from build123d import *

# Parameters (mm, degrees)
SKETCH2_W           = 46
SKETCH2_H           = 46
BOSS_EXTRUDE1_DEPTH = 5
SKETCH3_R           = 1.8
SKETCH3_R_2         = 2.5
CUT_EXTRUDE1_DEPTH  = 5
SKETCH4_R           = 4.1
CUT_EXTRUDE2_DEPTH  = 3
SKETCH5_W           = 4
SKETCH5_H           = 4
BOSS_EXTRUDE2_DEPTH = 3
SKETCH9_R           = 2
CUT_EXTRUDE6_DEPTH  = 6


with BuildPart() as part:
    # Sketch2 → Boss-Extrude1 (new body)
    with BuildSketch(Plane(origin=(0, 0, 0), x_dir=(1, 0, 0), z_dir=(0, 1, 0))):
        Rectangle(SKETCH2_W, SKETCH2_H)
    extrude(amount=BOSS_EXTRUDE1_DEPTH)

    # Sketch3 → Cut-Extrude1 (cut)
    with BuildSketch(Plane(origin=(0, 0, 0), x_dir=(1, 0, 0), z_dir=(0, 1, 0))):
        with Locations((-18.12, 19.125)):
            Circle(SKETCH3_R)
        with Locations((18.12, 19.125)):
            Circle(SKETCH3_R)
        with Locations((18.12, -19.125)):
            Circle(SKETCH3_R)
        with Locations((-18.12, -19.125)):
            Circle(SKETCH3_R)
        Circle(SKETCH3_R_2)
    extrude(amount=CUT_EXTRUDE1_DEPTH, mode=Mode.SUBTRACT)

    # Sketch4 → Cut-Extrude2 (cut)
    with BuildSketch(Plane(origin=(0, 0, 0), x_dir=(1, 0, 0), z_dir=(0, 1, 0))):
        Circle(SKETCH4_R)
    extrude(amount=CUT_EXTRUDE2_DEPTH, mode=Mode.SUBTRACT)

    # Sketch5 → Boss-Extrude2 (add)
    with BuildSketch(Plane(origin=(0, 0, 0), x_dir=(1, 0, 0), z_dir=(0, 1, 0))):
        with Locations((-5.7330026, 5.06948708)):
            Rectangle(SKETCH5_W, SKETCH5_H)
        with Locations((5.862376563, -4.939727226)):
            Rectangle(SKETCH5_W, SKETCH5_H)
    extrude(amount=-BOSS_EXTRUDE2_DEPTH)

    # Sketch9 → Cut-Extrude6 (cut, through all)
    with BuildSketch(Plane(origin=(0, 0, 0), x_dir=(1, 0, 0), z_dir=(0, 1, 0))):
        with Locations((-5.7330026, 20)):
            Circle(SKETCH9_R)
        with Locations((5.73, 20)):
            Circle(SKETCH9_R)
        with Locations((0, 20)):
            Circle(SKETCH9_R)
    extrude(amount=CUT_EXTRUDE6_DEPTH, mode=Mode.SUBTRACT)


solid = part.part
CAD build for the part. Positions are in the model's coordinates, mm. A direction names the side the tool comes from. Round coordinates to 2 decimals unless told otherwise and drop trailing zeros. Write each loop counter-clockwise with the first axis right and the second up, starting at its lowest first coordinate (ties: lowest second). Pieces come first, ordered by that corner, then holes. Notation, with made-up numbers: M -5.75,20 L 17.25,20 A21 cw 17.25,59 Z; hole C 18,23.25 d10. An arc over 180 degrees is marked long. Use a Markdown table: item, result. Add a question column.
1. Slice it at D-D on z = -1.5. Give the cut face in (x, y).
2. Drill centre lines: probe 1 along Z at (x, y) = (0, 1.85); probe 2 along X at (y, z) = (2, 0); probe 3 along Z at (x, y) = (-18.12, 1.55) (3 decimals). Where is each one in solid material? Low to high.
3. Slice it at A-A on x = 5.73. Give the cut face in (y, z).
4. Flat gauge pins, fed straight in: P1, Ø3, axis at x = 18.12, z = -19.125, coming from the -Y side; P2, Ø0.9, axis at x = -6.5, y = -1, coming from the -Z side; P3, Ø1.5, axis at y = -1, z = 5.5, coming from the +X side; P4, Ø0.9, axis at y = -1.5, z = -6, coming from the +X side. Where does each tip first touch, or does it go through?
5. Slice it at C-C on y = -2. Give the cut face in (x, z), then the cut area to 3 significant figures.
6. 3-axis set-ups, long thin cutter, end or side, ignore diameter. For faces 5 (the face through (6, -1, 2.94)), 6 (the face through (0, 2, 23)), 7 (the face through (-0.534, 1.479, -4.065)): which of +Z, -Z, +X, -X, +Y, -Y reach the whole face in a straight line?
7. Slice it at B-B on x = -18.12. Give the cut face in (y, z) (3 decimals).
8. Pull direction X, two halves, no side cores. Call faces 1 (the face through (7.862, -1, 5)), 2 (the face through (-2, 3, 2)), 3 (the face through (-7.733, -1, -5)), 4 (the face through (-6, -1, -7.069)): released by +X, released by -X, zero draft, split by the parting line, or undercut.
Reply:
| question | item | result |
|---|---|---|
| 1 | outline | M -23,0 L -3.82,0 L -3.82,3 L -2,3 L -2,5 L -23,5 Z; M 2,3 L 3.82,3 L 3.82,0 L 23,0 L 23,5 L 2,5 Z |
| 2 | probe 1 | z = -23 to -22, -18 to -4.1, 4.1 to 23 |
| 2 | probe 2 | x = -23 to -4.1, 4.1 to 23 |
| 2 | probe 3 | z = -23 to -20.925, -17.325 to 17.325, 20.925 to 23 |
| 3 | outline | M -3,2.94 L 0,2.94 L 0,-18 L 5,-18 L 5,23 L 0,23 L 0,6.94 L -3,6.94 Z; M 0,-23 L 5,-23 L 5,-22 L 0,-22 Z |
| 4 | P1 | passes through |
| 4 | P2 | stops at z = -7.07 |
| 4 | P3 | stops at x = 7.86 |
| 4 | P4 | stops at x = -3.73 |
| 5 | outline | M -7.73,-7.07 L -3.73,-7.07 L -3.73,-3.07 L -7.73,-3.07 Z; M 3.86,2.94 L 7.86,2.94 L 7.86,6.94 L 3.86,6.94 Z |
| 5 | area | 32.0 mm^2 |
| 6 | face 5 | -Z, +X, -X, -Y |
| 6 | face 6 | +Z, +X, -X, +Y, -Y |
| 6 | face 7 | -Y |
| 7 | outline | M 0,-23 L 5,-23 L 5,-20.925 L 0,-20.925 Z; M 0,-17.325 L 5,-17.325 L 5,17.325 L 0,17.325 Z; M 0,20.925 L 5,20.925 L 5,23 L 0,23 Z |
| 8 | face 1 | released by +X |
| 8 | face 2 | undercut |
| 8 | face 3 | released by -X |
| 8 | face 4 | zero draft |
